Geometry: final body of the model. Coordinates: model frame, mm. Face numbers are marked on the shaded views. Give positions to 0.01 mm unless a question says otherwise; leave off trailing zeros. Loops run counter-clockwise (first coordinate to the right, second up) from the corner with the lowest first, then second, coordinate; pieces in that order, holes last.
Autodesk Inventor part; units mm, degrees
ref_plane "YZ Plane" through (0, 0, 0) normal (1, 0, 0) x (0, 1, 0)
ref_plane "XZ Plane" through (0, 0, 0) normal (0, 1, 0) x (-1, 0, 0)
ref_plane "XY Plane" through (0, 0, 0) normal (0, 0, 1) x (1, 0, 0)
sketch "Sketch1" plane through (0, 0, 0) normal (0, 0, 1) x (1, 0, 0)
  line L0 (0, 0) -> (0, 50)
  line L1 (0, 50) -> (40, 50)
  line L2 (40, 50) -> (40, 20)
  line L3 (40, 20) -> (200, 20)
  line L4 (200, 20) -> (200, 0)
  line L5 (200, 0) -> (0, 0)
  line L6 (20, 50) -> (20, -1.8826)
  line L7 (20, -1.8826) -> (20, 0)
  circle A0 centre (20, 24.0587) radius 9.525
  dimension "d0" = 200
  dimension "d1" = 50
  dimension "d2" = 40
  dimension "d3" = 20
  dimension "d4" = 19.05
extrude "Extrusion1" add sketch "Sketch1" along normal blind 140 contours L0 L1 L6 A0 L5 | L6 A0 L1 L2 L3 L4 L5
fillet "Fillet1" radius 15 4 edges at (0, 50, 70) (40, 50, 70) (40, 20, 70) (0, 0, 70)
fillet "Fillet2" radius 20 2 edges at (200, 10, 140) (200, 10, 0)
fillet "Fillet3" radius 4 22 edges at (4.3933, 45.6067, 0) (0, 25, 0) (4.3933, 4.3933, 0) (97.4998, 0, 0) (194.1421, 0, 5.8579) (200, 0, 70) (194.1421, 0, 134.1421) (97.4998, 0, 140) (4.3933, 4.3933, 140) (0, 25, 140) (4.3933, 45.6067, 140) (20, 50, 140) (35.6067, 45.6067, 140) (40, 35, 140) (117.4998, 20, 140) (194.1421, 20, 134.1421) (200, 20, 70) (194.1421, 20, 5.8579) (117.4998, 20, 0) (40, 35, 0) (35.6067, 45.6067, 0) (20, 50, 0)
properties part number "foot rest EG26"
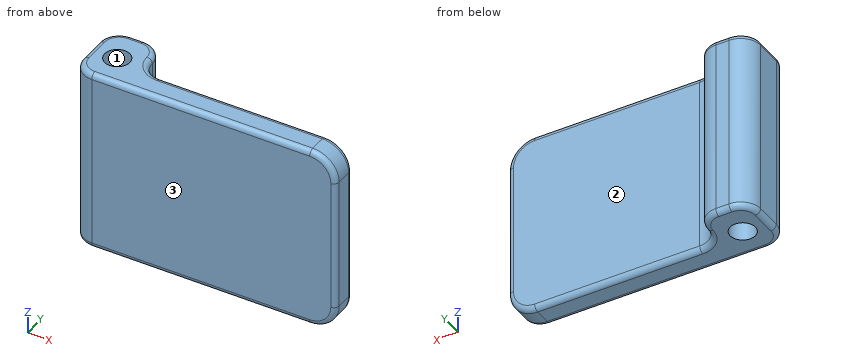
Item 1: Section query A-A on x = 20. Return loops of the section in (y, z).
Values follow:
outline: (0, 4) arc R4 ccw to (4, 0) - (14.53, 0) - (14.53, 140) - (4, 140) arc R4 ccw to (0, 136) - close; (33.58, 0) - (46, 0) arc R4 ccw to (50, 4) - (50, 136) arc R4 ccw to (46, 140) - (33.58, 140) - close
Item 2: Section query C-C on x = 138. Return loops of the section in (y, z).
Values follow:
outline: (0, 4) arc R4 ccw to (4, 0) - (16, 0) arc R4 ccw to (20, 4) - (20, 136) arc R4 ccw to (16, 140) - (4, 140) arc R4 ccw to (0, 136) - close
Item 3: Ray query, probe 1 along Y at (x, z) = (20, 73); probe 2 along Y at (x, z) = (112, 32.5); probe 3 along X at (y, z) = (21.5, 91.5). Return the intervals inside material, ascending.
Values follow:
probe 1: y = 0 to 14.53, 33.58 to 50
probe 2: y = 0 to 20
probe 3: x = 0 to 10.83, 29.17 to 48.46
Item 4: Pin query (flat end, axial travel): pin 1 (5 mm diameter, centred on x = 117, z = 45, fed in from -Y); pin 2 (1 mm diameter, centred on y = 36, z = 94, fed in from -X); pin 3 (4 mm diameter, centred on y = 10, z = 19.5, fed in from -X); pin 4 (5 mm diameter, centred on x = 140, z = 103.5, fed in from +Y). Return the tip coordinate at first contact, or that it passes through.
Values follow:
pin 1: stops at y = 0
pin 2: stops at x = 0.01
pin 3: stops at x = 0.3
pin 4: stops at y = 20
Item 5: Draft query along Y for the marked faces 1, 2 and 3. Return one class per face: +Y half, -Y half, draft (parallel to the pull), parting line (faces both ways), or undercut.
Values follow:
face 1: undercut
face 2: +Y half
face 3: -Y half
